```python
from build123d import *

# Parameters (mm, degrees)
SKETCH1_R           = 4.7625
SKETCH1_R_2         = 1.1303
BOSS_EXTRUDE1_DEPTH = 1.7145
SKETCH2_W           = 3.81
SKETCH2_H           = 2.54
CUT_EXTRUDE1_DEPTH  = 1.7145
SKETCH3_W           = 25.4
SKETCH3_H           = 9.525
CUT_EXTRUDE2_DEPTH  = 1.7145
FILLET1_R           = 0.762
FILLET2_R           = 0.762


with BuildPart() as part:
    # Sketch1 → Boss-Extrude1 (new body)
    with BuildSketch(Plane.XY):
        with BuildLine():
            Line((-30.1625, 9.245), (30.1625, 9.245))
            Line((30.1625, 9.245), (30.1625, 34.01))
            Line((30.1625, 34.01), (0, 34.01))
            ThreePointArc((0, 34.01), (-16.098329106, 29.958703243), (-28.361368091, 18.77))
            Line((-28.361368091, 18.77), (-30.1625, 18.77))
            Line((-30.1625, 18.77), (-30.1625, 9.245))
        make_face()
        with Locations((23.402088835, 27.025)):
            Circle(SKETCH1_R, mode=Mode.SUBTRACT)
        with Locations((-22.1869, 14.5155)):
            Circle(SKETCH1_R_2, mode=Mode.SUBTRACT)
        with Locations((14.813099914, 14.5155)):
            Circle(SKETCH1_R_2, mode=Mode.SUBTRACT)
        with Locations((27.212088835, 20.675)):
            Circle(SKETCH1_R_2, mode=Mode.SUBTRACT)
        with Locations((13.242088835, 29.565)):
            Circle(SKETCH1_R_2, mode=Mode.SUBTRACT)
    extrude(amount=BOSS_EXTRUDE1_DEPTH)

    # Sketch2 → Cut-Extrude1 (cut)
    with BuildSketch(Plane.XY.offset(1.7145)):
        with Locations((-1.644140797, 29.166672544)):
            Rectangle(SKETCH2_W, SKETCH2_H)
        with Locations((-1.644140797, 24.086672544)):
            Rectangle(SKETCH2_W, SKETCH2_H)
    extrude(amount=-CUT_EXTRUDE1_DEPTH, mode=Mode.SUBTRACT)

    # Sketch3 → Cut-Extrude2 (cut)
    with BuildSketch(Plane.XY.offset(1.7145)):
        with Locations((-3.686900043, 14.0075)):
            Rectangle(SKETCH3_W, SKETCH3_H)
    extrude(amount=-CUT_EXTRUDE2_DEPTH, mode=Mode.SUBTRACT)

    # Fillet1
    fillet1_edges = [part.edges().sort_by_distance(p)[0] for p in [
        (-28.361368091, 18.77, 0.85725),
        (30.1625, 34.01, 0.85725),
        (30.1625, 9.245, 0.85725),
        (-30.1625, 9.245, 0.85725),
        (-30.1625, 18.77, 0.85725),
        (-16.386900043, 9.245, 0.85725),
        (9.013099957, 9.245, 0.85725),
    ]]
    fillet(fillet1_edges, radius=FILLET1_R)

    # Fillet2
    fillet2_edges = [part.edges().sort_by_distance(p)[0] for p in [
        (-16.386900043, 18.77, 0.85725),
        (9.013099957, 18.77, 0.85725),
    ]]
    fillet(fillet2_edges, radius=FILLET2_R)


solid = part.part
```
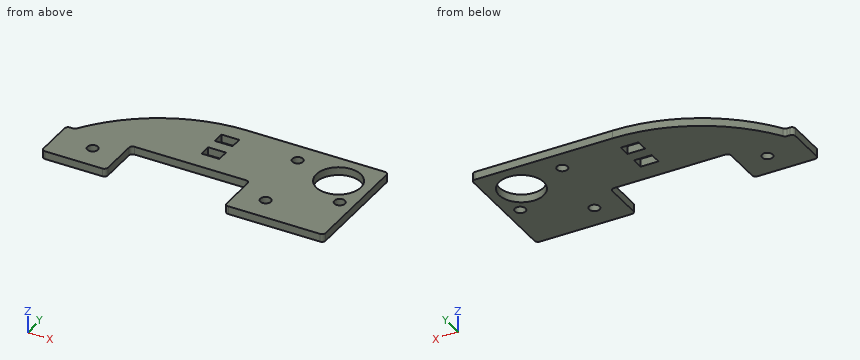
Source: CAD feature listing. Evaluate the final solid. Frame: model axes, mm. Round coordinates to 2 decimals unless told otherwise and drop trailing zeros. Write each loop counter-clockwise with the first axis right and the second up, starting at its lowest first coordinate (ties: lowest second). Pieces come first, ordered by that corner, then holes. Notation, with made-up numbers: M 5,24.5 L 27,24.5 A8 ccw 27,28.5 Z; hole C 40.25,-7.75 d7. An arc over 180 degrees is marked long. Answer as a JSON object with one key per item and string values. Group by question number.
(1) First-contact query: pin 1 (12 mm diameter, centred on x = 4, y = 18, fed in from +Z); pin 2 (1 mm diameter, centred on x = -9, z = 1, fed in from +Y); pin 3 (0.9 mm diameter, centred on y = 29, z = 0.5, fed in from -X). Flat tips, straight axial feed; report the tip coordinate or a pass-through.
(2) Ray query, line 1 (X direction, y = 17, z = 1.6); line 2 (Y direction, x = 0, z = 0.55); line 3 (X direction, y = 25.25, z = 0.25). Return the intervals inside material, ascending. Write a range as [from, to].
(3) Section query D-D on x = 6.5. Output: boundary loops of the cut face in (y, z).
(4) Section query A-A on y = 26.25. Output: boundary loops of the cut face in (x, z).
(5) Section query B-B on x = 23.5. Output: boundary loops of the cut face in (y, z) (1 decimal).
(6) Section query C-C on z = 0.8. State how many separate pieces and enclosed holes the cut face has, then the cut area to 3 significant figures.
Computed values:
{
 "1": {"pin 1": "z = 1.71", "pin 2": "y = 32.93", "pin 3": "x = -18.48"},
 "2": {"line 1": "[-30.16, -16.39], [9.01, 30.16]", "line 2": "[18.77, 22.82], [25.36, 27.9], [30.44, 34.01]", "line 3": "[-22.78, -3.55], [0.26, 18.98], [27.82, 30.16]"},
 "3": {"outline": "M 18.77,0 L 34.01,0 L 34.01,1.71 L 18.77,1.71 Z"},
 "4": {"outline": "M -21.62,0 L 18.7,0 L 18.7,1.71 L -21.62,1.71 Z; M 28.1,0 L 30.16,0 L 30.16,1.71 L 28.1,1.71 Z"},
 "5": {"outline": "M 9.2,0 L 22.3,0 L 22.3,1.7 L 9.2,1.7 Z; M 31.8,0 L 34,0 L 34,1.7 L 31.8,1.7 Z"},
 "6": {"separate pieces": "1", "enclosed holes": "7", "area": "989 mm^2"}
}
